The model under review builds one solid part; all positions refer to its coordinate system, in mm. A direction names the side the tool comes from. Give positions to 0.01 mm unless a question says otherwise; leave off trailing zeros. Order: outer loops, then holes, each group sorted by start corner. A loop starts at its lowest first (then second) coordinate and runs counter-clockwise, first axis right, second up.
```python
from build123d import *

# Parameters (mm, degrees)
F0_W     = 75
F0_H     = 130
F1_DEPTH = 40
F2_T     = -2.5
F4_DEPTH = 2.5
F5_W     = 18
F5_H     = 9
F6_DEPTH = 2.5
F8_DEPTH = 75


with BuildPart() as f1:
    # F0 (on Top) → F1 (new body)
    with BuildSketch(Plane.XY):
        with Locations((3.0821902634, 0)):
            Rectangle(F0_W, F0_H)
    extrude(amount=F1_DEPTH)

    # F2
    f2_openings = [f1.faces().sort_by_distance(p)[0] for p in [
        (3.08219, 0, 40),
    ]]
    offset(amount=F2_T, openings=f2_openings)

    # F3 (on face) → F4 (cut, through all)
    with BuildSketch(Plane.XZ.offset(65)):
        with BuildLine():
            Line((-18.0178097366, 40), (-24.8178097366, 40))
            Line((-24.8178097366, 40), (-24.8178097366, 15))
            ThreePointArc((-24.8178097366, 15), (-21.4178097366, 11.6), (-18.0178097366, 15))
            Line((-18.0178097366, 15), (-18.0178097366, 40))
        make_face()
        with BuildLine():
            Line((-8.2178097366, 40), (-15.0178097366, 40))
            Line((-15.0178097366, 40), (-15.0178097366, 15))
            ThreePointArc((-15.0178097366, 15), (-11.6178097366, 11.6), (-8.2178097366, 15))
            Line((-8.2178097366, 15), (-8.2178097366, 40))
        make_face()
        with BuildLine():
            Line((1.5821902634, 40), (-5.2178097366, 40))
            Line((-5.2178097366, 40), (-5.2178097366, 15))
            ThreePointArc((-5.2178097366, 15), (-1.8178097366, 11.6), (1.5821902634, 15))
            Line((1.5821902634, 15), (1.5821902634, 40))
        make_face()
        with BuildLine():
            Line((11.3821902634, 40), (4.5821902634, 40))
            Line((4.5821902634, 40), (4.5821902634, 15))
            ThreePointArc((4.5821902634, 15), (7.9821902634, 11.6), (11.3821902634, 15))
            Line((11.3821902634, 15), (11.3821902634, 40))
        make_face()
        with BuildLine():
            Line((21.1821902634, 15), (21.1821902634, 40))
            Line((21.1821902634, 40), (14.3821902634, 40))
            Line((14.3821902634, 40), (14.3821902634, 15))
            ThreePointArc((14.3821902634, 15), (17.7821902634, 11.6), (21.1821902634, 15))
        make_face()
        with BuildLine():
            Line((30.9821902634, 15), (30.9821902634, 40))
            Line((30.9821902634, 40), (24.1821902634, 40))
            Line((24.1821902634, 40), (24.1821902634, 15))
            ThreePointArc((24.1821902634, 15), (27.5821902634, 11.6), (30.9821902634, 15))
        make_face()
    extrude(amount=-F4_DEPTH, mode=Mode.SUBTRACT)

    # F5 (on face) → F6 (cut, through all)
    with BuildSketch(Plane(origin=(0, 65, 0), x_dir=(-1, 0, 0), z_dir=(0, 1, 0))):
        with Locations((-3.0821902634, 20)):
            Rectangle(F5_W, F5_H)
    extrude(amount=-F6_DEPTH, mode=Mode.SUBTRACT)

    # F7 (on face) → F8 (cut, through all)
    with BuildSketch(Plane.YZ.offset(40.5821902634)):
        with BuildLine():
            Line((-53.5, 8.790538609), (-53.5, 31.209461391))
            ThreePointArc((-53.5, 31.209461391), (-55.5, 33.209461391), (-57.5, 31.209461391))
            Line((-57.5, 31.209461391), (-57.5, 8.790538609))
            ThreePointArc((-57.5, 8.790538609), (-55.5, 6.790538609), (-53.5, 8.790538609))
        make_face()
        with BuildLine():
            Line((-29.5, 8.790538609), (-29.5, 31.209461391))
            ThreePointArc((-29.5, 31.209461391), (-31.5, 33.209461391), (-33.5, 31.209461391))
            Line((-33.5, 31.209461391), (-33.5, 8.790538609))
            ThreePointArc((-33.5, 8.790538609), (-31.5, 6.790538609), (-29.5, 8.790538609))
        make_face()
        with BuildLine():
            Line((-17.5, 8.790538609), (-17.5, 31.209461391))
            ThreePointArc((-17.5, 31.209461391), (-19.5, 33.209461391), (-21.5, 31.209461391))
            Line((-21.5, 31.209461391), (-21.5, 8.790538609))
            ThreePointArc((-21.5, 8.790538609), (-19.5, 6.790538609), (-17.5, 8.790538609))
        make_face()
        with BuildLine():
            Line((-5.5, 8.790538609), (-5.5, 31.209461391))
            ThreePointArc((-5.5, 31.209461391), (-7.5, 33.209461391), (-9.5, 31.209461391))
            Line((-9.5, 31.209461391), (-9.5, 8.790538609))
            ThreePointArc((-9.5, 8.790538609), (-7.5, 6.790538609), (-5.5, 8.790538609))
        make_face()
        with BuildLine():
            Line((6.5, 8.790538609), (6.5, 31.209461391))
            ThreePointArc((6.5, 31.209461391), (4.5, 33.209461391), (2.5, 31.209461391))
            Line((2.5, 31.209461391), (2.5, 8.790538609))
            ThreePointArc((2.5, 8.790538609), (4.5, 6.790538609), (6.5, 8.790538609))
        make_face()
        with BuildLine():
            Line((18.5, 8.790538609), (18.5, 31.209461391))
            ThreePointArc((18.5, 31.209461391), (16.5, 33.209461391), (14.5, 31.209461391))
            Line((14.5, 31.209461391), (14.5, 8.790538609))
            ThreePointArc((14.5, 8.790538609), (16.5, 6.790538609), (18.5, 8.790538609))
        make_face()
        with BuildLine():
            Line((30.5, 8.790538609), (30.5, 31.209461391))
            ThreePointArc((30.5, 31.209461391), (28.5, 33.209461391), (26.5, 31.209461391))
            Line((26.5, 31.209461391), (26.5, 8.790538609))
            ThreePointArc((26.5, 8.790538609), (28.5, 6.790538609), (30.5, 8.790538609))
        make_face()
        with BuildLine():
            Line((42.5, 8.790538609), (42.5, 31.209461391))
            ThreePointArc((42.5, 31.209461391), (40.5, 33.209461391), (38.5, 31.209461391))
            Line((38.5, 31.209461391), (38.5, 8.790538609))
            ThreePointArc((38.5, 8.790538609), (40.5, 6.790538609), (42.5, 8.790538609))
        make_face()
        with BuildLine():
            Line((54.5, 8.790538609), (54.5, 31.209461391))
            ThreePointArc((54.5, 31.209461391), (52.5, 33.209461391), (50.5, 31.209461391))
            Line((50.5, 31.209461391), (50.5, 8.790538609))
            ThreePointArc((50.5, 8.790538609), (52.5, 6.790538609), (54.5, 8.790538609))
        make_face()
        with BuildLine():
            Line((-41.5, 8.790538609), (-41.5, 31.209461391))
            ThreePointArc((-41.5, 31.209461391), (-43.5, 33.209461391), (-45.5, 31.209461391))
            Line((-45.5, 31.209461391), (-45.5, 8.790538609))
            ThreePointArc((-45.5, 8.790538609), (-43.5, 6.790538609), (-41.5, 8.790538609))
        make_face()
    extrude(amount=-F8_DEPTH, mode=Mode.SUBTRACT)


solid = f1.part
```
1. Take a section at B-B (y = -55.5). Write out the cut boundary in (x, z), and give its area (3 significant figures).
2. Insertion check: pin 1 (1.5 mm diameter, centred on x = 27, y = -32, fed in from -Z). The pin has a flat end and moves straight along its axis. Give the tip position at first contact, or say it passes through.
3. Draft analysis for pull direction X (two halves, no side actions). For faces 1 (the flat face through (11.382, -64, 27)), 2 (the flat face through (-33, -17.5, 20)), state which applies: pulls with the +X half, pulls with the -X half, needs draft (parallel to the pull), parting line crosses it, or undercut.
4. For faces 3 (the flat face through (13, -64, 40)), 4 (the flat face through (-33, -5.5, 20)), 5 (the flat face through (-18.018, -64, 27)), list the 3-axis set-ups (+Z, -Z, +X, -X, +Y, -Y) from which the entire face can be reached by the end or side of a thin tool; tool diameter is ignored.
5. Take a section at C-C (x = -1.5). Write out the cut boundary in (y, z).
6. Take a section at D-D (z = 4). Write out the cut boundary in (x, y), and give its area (3 significant figures).
7. Take a section at A-A (z = 35.5). Count the separate pieces of the cut face and the enclosed holes in it, and give its area (3 significant figures).
8. To check wall thickness, follow line 1 (Y direction, x = 17, z = 9); line 2 (X direction, y = 19.5, z = 3); line 3 (Y direction, x = -10.5, z = 12). State the ranges of each line that lie inside material, in increasing order.
Answer:
1. outline: (-34.42, 0) - (40.58, 0) - (40.58, 6.79) - (38.08, 6.79) - (38.08, 2.5) - (-31.92, 2.5) - (-31.92, 6.79) - (-34.42, 6.79) - close; (-34.42, 33.21) - (-31.92, 33.21) - (-31.92, 40) - (-34.42, 40) - close; (38.08, 33.21) - (40.58, 33.21) - (40.58, 40) - (38.08, 40) - close
1. area: 243 mm2
2. pin 1: stops at z = 0
3. face 1: undercut
3. face 2: needs draft
4. face 3: +Z, +X, -X, +Y, -Y
4. face 4: +X, -X
4. face 5: +Z, -Y
5. outline: (-65, 0) - (65, 0) - (65, 15.5) - (62.5, 15.5) - (62.5, 2.5) - (-62.5, 2.5) - (-62.5, 11.61) - (-65, 11.61) - close; (62.5, 24.5) - (65, 24.5) - (65, 40) - (62.5, 40) - close
6. outline: (-34.42, -65) - (40.58, -65) - (40.58, 65) - (-34.42, 65) - close; hole (-31.92, -62.5) - (38.08, -62.5) - (38.08, 62.5) - (-31.92, 62.5) - close
6. area: 1,000 mm2
7. separate pieces: 6
7. enclosed holes: 0
7. area: 898 mm2
8. line 1: y = -65 to -62.5, 62.5 to 65
8. line 2: x = -34.42 to -31.92, 38.08 to 40.58
8. line 3: y = 62.5 to 65
